Autodesk Inventor part; units mm, degrees
ref_plane "YZ Plane" through (0, 0, 0) normal (1, 0, 0) x (0, 1, 0)
ref_plane "XZ Plane" through (0, 0, 0) normal (0, 1, 0) x (-1, 0, 0)
ref_plane "XY Plane" through (0, 0, 0) normal (0, 0, 1) x (1, 0, 0)
sketch "Platine" plane through (0, 0, 0) normal (0, 0, 1) x (1, 0, 0)
  line L0 (-25, -19.16) -> (25, -19.16)
  line L1 (25, -19.16) -> (25, 30.84)
  line L2 (25, 30.84) -> (-25, 30.84)
  line L3 (-25, 30.84) -> (-25, -19.16)
  line L4 (-25, -19.16) -> (25, 30.84)
  line L5 (25, -19.16) -> (-25, 30.84)
  line L6 (-31, -2.16) -> (-9, -2.16)
  line L7 (-9, -2.16) -> (-9, 13.84)
  line L8 (-9, 13.84) -> (-31, 13.84)
  line L9 (-31, 13.84) -> (-31, -2.16)
  line L10 (29, -9.76) -> (15, -9.76)
  line L11 (15, -9.76) -> (15, -0.21)
  line L12 (15, -0.21) -> (29, -0.21)
  line L13 (29, -0.21) -> (29, -9.76)
  line L14 (15, 7.84) -> (29, 7.84)
  line L15 (29, 7.84) -> (29, 18)
  line L16 (29, 18) -> (15, 18)
  line L17 (15, 18) -> (15, 7.84)
  circle A0 centre (-20, 25.84) radius 1.5
  circle A1 centre (20, -14.16) radius 1.5
  line L18 (-31, 32.4529) -> (-31, -19) construction
  line L19 (29, 40.2658) -> (29, -31.3692) construction
  line L20 (-20, 25.84) -> (20, 25.84) construction
  line L21 (20, 25.84) -> (20, -14.16) construction
  line L22 (20, -14.16) -> (-20, -14.16) construction
  line L23 (-20, -14.16) -> (-20, 25.84) construction
  circle A2 centre (20, 25.84) radius 1.5
  circle A3 centre (-20, -14.16) radius 1.5
  point P0 (0, 0)
  point P1 (0, 5.84)
  dimension "d0" = 50
  dimension "d1" = 50
  dimension "d2" = 22
  dimension "d3" = 16
  dimension "d4" = 17
  dimension "d6" = 14
  dimension "d7" = 9.55
  dimension "d8" = 9.4
  dimension "d10" = 10.16
  dimension "d11" = 14
  dimension "d12" = 27
  dimension "d14" = 3
  dimension "d15" = 5
  dimension "d16" = 5
  dimension "d17" = 5
  dimension "d18" = 5
  dimension "d19" = 18
  dimension "d127" = 6
  dimension "d128" = 4
  dimension "d129" = 25
extrude "Platinengeometrie" add sketch "Platine" against normal blind 2 contours L4 A3 L5 L11 L10 A1 L0 | L3 L6 L7 L8 L5 A0 L4 A3 | L5 A1 L10 L1 | L3 L8 L7 L6 | A3 L4 | L4 A3 | L10 L5 L11 L12 L1 | A1 L5 | L5 A1 | L12 L11 L5 L4 A2 L1 L16 L17 L14 | L10 L11 L5 | L2 L4 A2 L5 A0 | L14 L17 L16 L1 | A0 L5 | L5 A0 | A2 L4 | L4 A2
extrude "MEBP 8-8G" add sketch "Platine" along normal blind 13.5 contours L6 L9 L8 L3 | L3 L8 L7 L6
extrude "HEBW21" add sketch "Platine" along normal blind 11 contours L10 L5 L11 L12 L1 | L1 L12 L13 L10 | L10 L11 L5
extrude "PSS 254/4W" add sketch "Platine" along normal blind 5 contours L14 L17 L16 L1 | L1 L16 L15 L14
extrude "Extrusion9" cut sketch "Platine" against normal up to next contours A1 L5 | L5 A1 | A0 L5 | L5 A0
equation "\"d136\" = d18"
properties part number "PCB-Model"
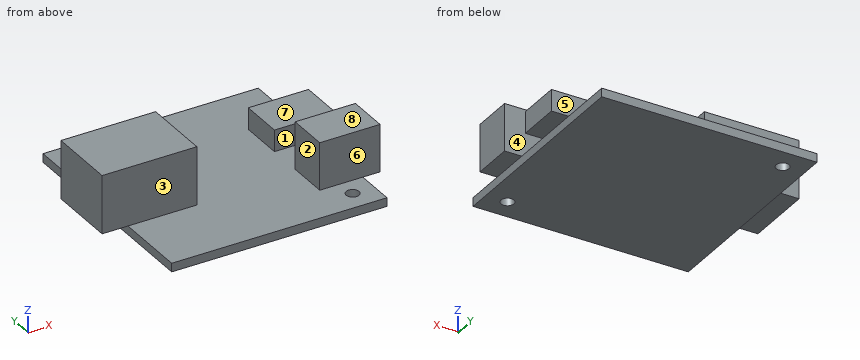
Verification items for the finished model (mm, model axes). Face numbers are marked on the shaded views. A direction names the side the tool comes from. Round coordinates to 2 decimals unless told otherwise and drop trailing zeros. Order: outer loops, then holes, each group sorted by start corner. A loop starts at its lowest first (then second) coordinate and runs counter-clockwise, first axis right, second up. Notation, with made-up numbers: (28, 84.5) - (87, 84.5) arc R23 cw to (87, 120.5) - close; hole circle Ø8 at (63.25, 43.25). An arc over 180 degrees is marked (long way). Use CSV: the item, a comma, the result in double quotes. Start each with the question number.
1) Mould release check, pull along Y, two halves, no side actions. Record for the marked faces 1, 2 and 3: +Y half, -Y half, draft (parallel to the pull), parting line (faces both ways), or undercut.
2) Thickness scan on L1, parallel to X at y = -14.16, z = -0.9; L2, parallel to Y at x = 22.5, z = 4.5; L3, parallel to X at y = 25.84, z = -0.55. Record the ranges inside material, lowest first.
3) Access from +Z, -Z, +X, -X, +Y, -Y to the whole of each face (thin tool, end or side, straight path). Record for the marked faces 4, 5, 6, 7 and 8.
4) Go/stop test with flat-tipped pins: P1, Ø3, axis at x = 24, y = -7, coming from the +Z side; P2, Ø25, axis at x = 6.5, y = 16.5, coming from the +Z side; P3, Ø0.6, axis at y = 17.5, z = -0.5, coming from the -X side. Record where each tip stops, or that it passes through.
5) Section check B-B, the plane z = 7.5. Record the cut outline in (x, y).
6) Section check A-A, the plane y = -14.16. Record the cut outline in (x, z).
7) Section check D-D, the plane z = 4.25. Record the cut outline in (x, y), plus the area to 3 significant figures.
8) Section check C-C, the plane x = 20. Record the cut outline in (y, z), plus the area to 3 significant figures.
Answers:
1,face 1,"undercut"
1,face 2,"draft"
1,face 3,"-Y half"
2,L1,"x = -25 to 18.5, 21.5 to 25"
2,L2,"y = -9.76 to -0.21, 7.84 to 18"
2,L3,"x = -25 to -21.5, -18.5 to 25"
3,face 4,"+Z, +X"
3,face 5,"+Z, +X, -X, +Y"
3,face 6,"+Z, +X, -X, -Y"
3,face 7,"+Z, +X, +Y"
3,face 8,"+Z, +X, +Y, -Y"
4,P1,"stops at z = 11"
4,P2,"stops at z = 5"
4,P3,"stops at x = -25"
5,outline,"(-31, -2.16) - (-9, -2.16) - (-9, 13.84) - (-31, 13.84) - close; (15, -9.76) - (29, -9.76) - (29, -0.21) - (15, -0.21) - close"
6,outline,"(-25, -2) - (18.5, -2) - (18.5, 0) - (-25, 0) - close; (21.5, -2) - (25, -2) - (25, 0) - (21.5, 0) - close"
7,outline,"(-31, -2.16) - (-9, -2.16) - (-9, 13.84) - (-31, 13.84) - close; (15, -9.76) - (29, -9.76) - (29, -0.21) - (15, -0.21) - close; (15, 7.84) - (29, 7.84) - (29, 18) - (15, 18) - close"
7,area,"628 mm²"
8,outline,"(-19.16, -2) - (-15.66, -2) - (-15.66, 0) - (-19.16, 0) - close; (-12.66, -2) - (30.84, -2) - (30.84, 0) - (18, 0) - (18, 5) - (7.84, 5) - (7.84, 0) - (-0.21, 0) - (-0.21, 11) - (-9.76, 11) - (-9.76, 0) - (-12.66, 0) - close"
8,area,"250 mm²"
